Work out the finished part from the listing and answer in its coordinate system (mm). A direction names the side the tool comes from. Round coordinates to 2 decimals unless told otherwise and drop trailing zeros. Order: outer loops, then holes, each group sorted by start corner. A loop starts at its lowest first (then second) coordinate and runs counter-clockwise, first axis right, second up. Notation, with made-up numbers: (78, -29.5) - (129, -29.5) arc R31 cw to (129, 9.5) - close; hole circle Ø4 at (-11, 10.25). An arc over 180 degrees is marked (long way). Use one line per item in the form item = value. Start each with the question number.
Q1. Given P1, Ø5, axis at x = 28.5, y = 4, coming from the +Z side; P2, Ø4, axis at x = 31, y = 4, coming from the -Z side; P3, Ø2, axis at y = 9, z = -23, coming from the -X side, each flat-ended and moving along its own axis, determine where each tip first touches the part or whether it passes through.
Q2. The part is cut by section C-C on y = 8. Determine the outline of the cut face in (x, z) (3 decimals).
Q3. The part is cut by section A-A on x = 0. Determine the outline of the cut face in (y, z) (3 decimals), plus the area to 3 significant figures.
Q4. The part is cut by section B-B on z = 0. Determine the outline of the cut face in (x, y) (3 decimals).
Q5. For a pull along X with two mould halves and no side action, classify faces 1 (the flat face through (-1, 12.7, 12)), 2 (the cylindrical face through (-0.69, 6.26, -3.1)), 3 (the cylindrical face through (-41.27, 6.26, 0.14)), 4 (the conical face through (-13.19, 0.12, 59.38)) as +X half, -X half, draft (parallel to the pull), parting line (faces both ways), or undercut.
Q6. Which of the six approach directions +Z, -Z, +X, -X, +Y, -Y give full straight-line access (tool end or side, diameter ignored) to faces 5 (the cylindrical face through (-57.095, 8.854, -2.513)), 6 (the flat face through (-1, 0, 13))?
Q7. Find the intervals of material crossed by line 1 (Z direction, x = 0, y = 3.75) (3 decimals); line 2 (Z direction, x = 0, y = 10) (3 decimals); line 3 (Y direction, x = -5, z = 57.5), in increasing order. Write a range as [from, to].
from build123d import *

# Parameters (mm, degrees)
SKETCH1_R           = 63.246
BOSS_EXTRUDE1_DEPTH = 6.35
SKETCH2_R           = 57.15
BOSS_EXTRUDE2_DEPTH = 6.35
CHAMFER1_SIZE       = 1.27
SKETCH4_R           = 3.175
CUT_EXTRUDE1_DEPTH  = 13.7
CHAMFER2_SIZE       = 2.54


with BuildPart() as part:
    # Sketch1 → Boss-Extrude1 (new body)
    with BuildSketch(Plane(origin=(0, 0, 0), x_dir=(1, 0, 0), z_dir=(0, 1, 0))):
        Circle(SKETCH1_R)
    extrude(amount=BOSS_EXTRUDE1_DEPTH)

    # Sketch2 → Boss-Extrude2 (add)
    with BuildSketch(Plane(origin=(0, 6.35, 0), x_dir=(1, 0, 0), z_dir=(0, 1, 0))):
        Circle(SKETCH2_R)
    extrude(amount=BOSS_EXTRUDE2_DEPTH)

    # Chamfer1
    chamfer1_edges = [part.edges().sort_by_distance(p)[0] for p in [
        (-57.15, 12.7, 0),
    ]]
    chamfer(chamfer1_edges, length=CHAMFER1_SIZE)

    # Sketch4 → Cut-Extrude1 (cut, through all)
    with BuildSketch(Plane.XZ):
        with Locations((-38.1, 0)):
            Circle(SKETCH4_R)
        Circle(SKETCH4_R)
        with Locations((38.1, 0)):
            Circle(SKETCH4_R)
    extrude(amount=-CUT_EXTRUDE1_DEPTH, mode=Mode.SUBTRACT)

    # Chamfer2
    chamfer2_edges = [part.edges().sort_by_distance(p)[0] for p in [
        (-63.246, 0, 0),
    ]]
    chamfer(chamfer2_edges, length=CHAMFER2_SIZE)


solid = part.part
Found:
q1.P1 = 57.65
q1.P2 = -56.21
q1.P3 = -52.75
q2.outline = circle Ø114.3 at (0, 0); hole circle Ø6.35 at (-38.1, 0); hole circle Ø6.35 at (0, 0); hole circle Ø6.35 at (38.1, 0)
q3.outline = (0, -60.706) - (2.54, -63.246) - (6.35, -63.246) - (6.35, -57.15) - (11.43, -57.15) - (12.7, -55.88) - (12.7, -3.175) - (0, -3.175) - close; (0, 3.175) - (12.7, 3.175) - (12.7, 55.88) - (11.43, 57.15) - (6.35, 57.15) - (6.35, 63.246) - (2.54, 63.246) - (0, 60.706) - close
q3.area = 1,440 mm²
q4.outline = (-63.246, 2.54) - (-60.706, 0) - (-41.275, 0) - (-41.275, 12.7) - (-55.88, 12.7) - (-57.15, 11.43) - (-57.15, 6.35) - (-63.246, 6.35) - close; (-34.925, 0) - (-3.175, 0) - (-3.175, 12.7) - (-34.925, 12.7) - close; (3.175, 0) - (34.925, 0) - (34.925, 12.7) - (3.175, 12.7) - close; (41.275, 0) - (60.706, 0) - (63.246, 2.54) - (63.246, 6.35) - (57.15, 6.35) - (57.15, 11.43) - (55.88, 12.7) - (41.275, 12.7) - close
q5.face_1 = draft
q5.face_2 = undercut
q5.face_3 = undercut
q5.face_4 = parting line
q6.face_5 = +Y
q6.face_6 = +Z, -Z, +X, -X, -Y
q7.line_1 = [-63.246, -3.175], [3.175, 63.246]
q7.line_2 = [-57.15, -3.175], [3.175, 57.15]
q7.line_3 = [0, 6.35]
